```python
from build123d import *

# Parameters (mm, degrees)
SKETCH1_W                = 502.069989
SKETCH1_H                = 502.069989
SKETCH1_W_2              = 476.669989
SKETCH1_H_2              = 476.669989
EXTRUDE1_DEPTH           = 6.35
SKETCH2_W                = 502.069989
SKETCH2_H                = 502.069989
SKETCH2_W_2              = 451.269989
SKETCH2_H_2              = 451.269989
EXTRUDE2_DEPTH           = 3.175
SKETCH7_W                = 6.35
SKETCH7_H                = 502.069989
EXTRUDE3_DEPTH           = 9.525
F_5_16_CLEARANCE_HOLE1_D = 8.72998
SKETCH8_W                = 19.05
SKETCH8_H                = 25.4
CUT_EXTRUDE1_DEPTH       = 6.35
LPATTERN1_COUNT          = 2
LPATTERN1_PITCH          = 101.6
MIRROR2_COPY_1_SKETCH_W  = 19.05
MIRROR2_COPY_1_SKETCH_H  = 25.4
MIRROR2_COPY_1_DEPTH     = 6.35
EXTRUDE4_DEPTH           = 360.591332428
FILLET1_R                = 3.175


with BuildPart() as part:
    # Sketch1 → Extrude1 (new body)
    with BuildSketch(Plane.XY):
        Rectangle(SKETCH1_W, SKETCH1_H)
        Rectangle(SKETCH1_W_2, SKETCH1_H_2, mode=Mode.SUBTRACT)
    extrude(amount=-EXTRUDE1_DEPTH)

    # Sketch2 → Extrude2 (add)
    with BuildSketch(Plane.XY):
        Rectangle(SKETCH2_W, SKETCH2_H)
        Rectangle(SKETCH2_W_2, SKETCH2_H_2, mode=Mode.SUBTRACT)
    extrude(amount=EXTRUDE2_DEPTH)

    # Sketch7 → Extrude3 (add)
    with BuildSketch(Plane.XY.offset(3.175)):
        with Locations((-254.2099945, 0)):
            Rectangle(SKETCH7_W, SKETCH7_H)
    extrude3 = extrude(amount=-EXTRUDE3_DEPTH)

    # Mirror1: Extrude3 across plane
    add(extrude3.mirror(Plane(origin=(0, 0, 0), x_dir=(0, 0, 1), z_dir=(1, 0, 0))))

    # 5/16 Clearance Hole1 (through all)
    with Locations(Plane.XY.offset(3.175)):
        with Locations((251.0349945, -50.8), (251.0349945, 50.8), (-251.0349945, -50.8), (-251.0349945, 50.8)):
            Hole(F_5_16_CLEARANCE_HOLE1_D / 2)

    # Sketch8 → Cut-Extrude1 (cut)
    with BuildSketch(Plane(origin=(0, 0, -6.35), x_dir=(-1, 0, 0), z_dir=(0, 0, -1))):
        with Locations((247.8599945, 50.8)):
            Rectangle(SKETCH8_W, SKETCH8_H)
    cut_extrude1 = extrude(amount=-CUT_EXTRUDE1_DEPTH, mode=Mode.SUBTRACT)

    # LPattern1: Cut-Extrude1 ×2
    with Locations(*[(0, -i * LPATTERN1_PITCH, 0) for i in range(1, LPATTERN1_COUNT)]):
        add(cut_extrude1, mode=Mode.SUBTRACT)

    # Mirror2: Cut-Extrude1 across plane
    add(cut_extrude1.mirror(Plane(origin=(0, 0, 0), x_dir=(0, 0, 1), z_dir=(1, 0, 0))), mode=Mode.SUBTRACT)

    # Mirror2 copy 1 sketch → Mirror2 copy 1 (cut)
    with BuildSketch(Plane(origin=(0, -101.6, -6.35), x_dir=(1, 0, 0), z_dir=(0, 0, -1))):
        with Locations((247.8599945, -50.8)):
            Rectangle(MIRROR2_COPY_1_SKETCH_W, MIRROR2_COPY_1_SKETCH_H)
    extrude(amount=-MIRROR2_COPY_1_DEPTH, mode=Mode.SUBTRACT)

    # Sketch9 → Extrude4 (cut, through all)
    with BuildSketch(Plane(origin=(0, 0, 0), x_dir=(-1, 0, 0), z_dir=(0, 0, -1))):
        with BuildLine():
            Line((-238.3349945, 238.3349945), (-235.1599945, 238.3349945))
            Line((-235.1599945, 238.3349945), (-235.1599945, 235.1599945))
            ThreePointArc((-235.1599945, 235.1599945), (-240.58005853, 232.91493047), (-238.3349945, 238.3349945))
        make_face()
        with BuildLine():
            Line((235.1599945, 238.3349945), (235.1599945, 235.1599945))
            ThreePointArc((235.1599945, 235.1599945), (240.58005853, 232.91493047), (238.3349945, 238.3349945))
            Line((238.3349945, 238.3349945), (235.1599945, 238.3349945))
        make_face()
        with BuildLine():
            Line((238.3349945, -238.3349945), (235.1599945, -238.3349945))
            Line((235.1599945, -238.3349945), (235.1599945, -235.1599945))
            ThreePointArc((235.1599945, -235.1599945), (240.58005853, -232.91493047), (238.3349945, -238.3349945))
        make_face()
        with BuildLine():
            Line((-235.1599945, -238.3349945), (-235.1599945, -235.1599945))
            ThreePointArc((-235.1599945, -235.1599945), (-240.58005853, -232.91493047), (-238.3349945, -238.3349945))
            Line((-238.3349945, -238.3349945), (-235.1599945, -238.3349945))
        make_face()
    extrude(amount=EXTRUDE4_DEPTH, mode=Mode.SUBTRACT)

    # Fillet1
    fillet1_edges = [part.edges().sort_by_distance(p)[0] for p in [
        (-225.6349945, 225.6349945, 1.5875),
        (-225.6349945, -225.6349945, 1.5875),
        (225.6349945, -225.6349945, 1.5875),
        (225.6349945, 225.6349945, 1.5875),
    ]]
    fillet(fillet1_edges, radius=FILLET1_R)


solid = part.part
```
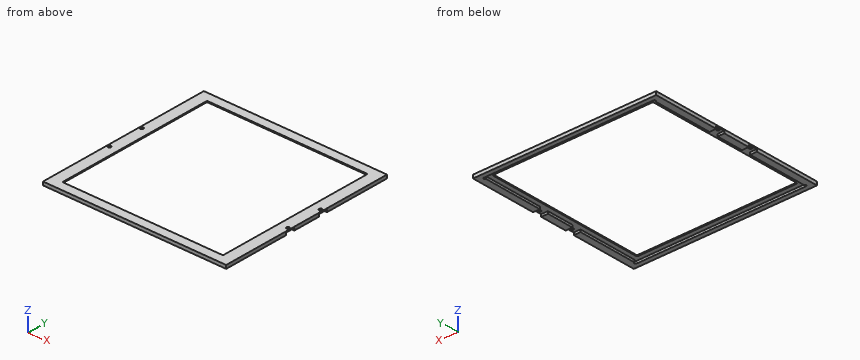
Could you check a few things on this model? Use its own coordinates, in mm. Round coordinates to 2 decimals unless told otherwise and drop trailing zeros. Loops run counter-clockwise (first coordinate to the right, second up) from the corner with the lowest first, then second, coordinate; pieces in that order, holes last. Notation, with made-up numbers: (27.5, -28) - (64.5, -28) arc R23 cw to (64.5, -2) - close; hole circle Ø2 at (8, -38.5). An arc over 180 degrees is marked (long way). Answer in a Markdown table with one row per item. Add a question column.
(1) If we section it at B-B (x = -146): Please give me the cut outline in (y, z) (3 decimals).
(2) If we section it at C-C (z = -4.5): Please give me the cut outline in (x, y) (3 decimals).
(3) I need wall thicknesses on line 1 along X through (y, z) = (-174, -0.75) (3 decimals); line 2 along Y through (x, z) = (143.5, -4) (3 decimals); line 3 along Y through (x, z) = (211, 1.5) (3 decimals). Which ranges of each line are inside material? Lowest first, please.
(4) If we section it at A-A (y = -203): Please give me the cut outline in (x, z) (3 decimals).
Model answer:
| question | item | result |
|---|---|---|
| 1 | outline | (-251.035, -6.35) - (-238.335, -6.35) - (-238.335, 0) - (-225.635, 0) - (-225.635, 3.175) - (-251.035, 3.175) - close; (225.635, 0) - (238.335, 0) - (238.335, -6.35) - (251.035, -6.35) - (251.035, 3.175) - (225.635, 3.175) - close |
| 2 | outline | (-257.385, -251.035) - (257.385, -251.035) - (257.385, -63.5) - (238.335, -63.5) - (238.335, -231.985) arc R3.175 cw to (238.335, -238.335) - (-238.335, -238.335) arc R3.175 cw to (-238.335, -231.985) - (-238.335, -63.5) - (-257.385, -63.5) - close; (-257.385, -38.1) - (-238.335, -38.1) - (-238.335, 38.1) - (-257.385, 38.1) - close; (-257.385, 63.5) - (-238.335, 63.5) - (-238.335, 231.985) arc R3.175 cw to (-238.335, 238.335) - (238.335, 238.335) arc R3.175 cw to (238.335, 231.985) - (238.335, 63.5) - (257.385, 63.5) - (257.385, 251.035) - (-257.385, 251.035) - close; (238.335, -38.1) - (257.385, -38.1) - (257.385, 38.1) - (238.335, 38.1) - close |
| 3 | line 1 | x = -257.385 to -238.335, 238.335 to 257.385 |
| 3 | line 2 | y = -251.035 to -238.335, 238.335 to 251.035 |
| 3 | line 3 | y = -251.035 to -225.635, 225.635 to 251.035 |
| 4 | outline | (-257.385, -6.35) - (-238.335, -6.35) - (-238.335, 0) - (-225.635, 0) - (-225.635, 3.175) - (-257.385, 3.175) - close; (225.635, 0) - (238.335, 0) - (238.335, -6.35) - (257.385, -6.35) - (257.385, 3.175) - (225.635, 3.175) - close |
